Build history of the part. All positions in model axes, mm. Give positions to 0.01 mm unless a question says otherwise; leave off trailing zeros. Loops run counter-clockwise (first coordinate to the right, second up) from the corner with the lowest first, then second, coordinate; pieces in that order, holes last. Notation, with made-up numbers: M -13,6.5 L 20,6.5 A23 ccw 20,14.5 Z; hole C 89.5,-14 d8. An arc over 180 degrees is marked long. Answer as a JSON object with one key per item and string values. Group by question number.
1. Slice it at C-C (y = -11). List the corners of the cut face in (x, z), then the cut area to 3 significant figures.
2. Slice it at A-A (x = 0). List the corners of the cut face in (y, z), then the cut area to 3 significant figures.
3. Drop flat-ended pins along their axis: pin 1 Ø2 at (y, z) = (0.5, 2) entering from +X; pin 2 Ø2 at (y, z) = (-28, 4) entering from +X; pin 3 Ø3 at (x, y) = (-13, 36) entering from +Z; pin 4 Ø3 at (y, z) = (-46, 1) entering from -X. Give the stop position or say it passes through.
4. Slice it at D-D (y = -45). List the corners of the cut face in (x, z), then the cut area to 3 significant figures.
5. Slice it at B-B (z = 5.1). List the corners of the cut face in (x, y).
6. Drill centre lines: line 1 along Y through (x, z) = (0, 3.4); line 2 along Y through (x, z) = (7.5, 0.25); line 3 along X through (y, z) = (-31.5, 2.9). Where is each one in solid material? Low to high. Write a range as [from, to].
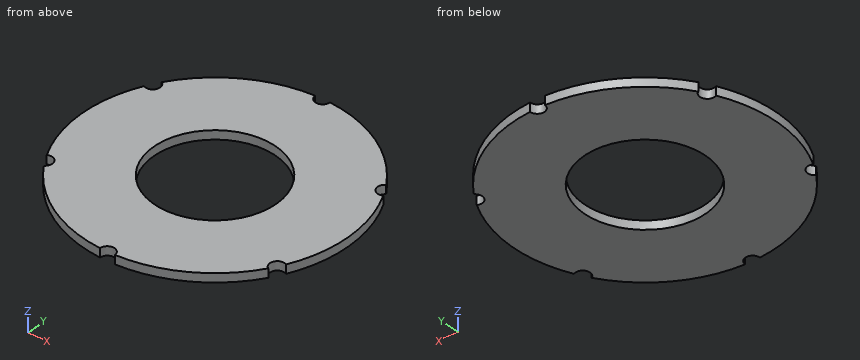
from build123d import *

# Parameters (mm, degrees)
SKETCH1_R                  = 90
SKETCH1_R_2                = 41.5
BOSS_EXTRUDE1_DEPTH        = 6
F_10_0MM_DOWEL_HOLE1_D     = 10
F_10_0MM_DOWEL_HOLE1_DEPTH = 9.906
F_10_0MM_DOWEL_HOLE1_TIP   = 3.004303095


with BuildPart() as part:
    # Sketch1 → Boss-Extrude1 (new body)
    with BuildSketch(Plane.XY):
        Circle(SKETCH1_R)
        Circle(SKETCH1_R_2, mode=Mode.SUBTRACT)
    extrude(amount=BOSS_EXTRUDE1_DEPTH)

    # Ø10.0mm Dowel Hole1
    with Locations(Plane(origin=(0, 0, 0), x_dir=(-1, 0, 0), z_dir=(0, 0, -1))):
        with Locations((-77.942286341, 45), (-77.942286341, -45), (0, -90), (77.942286341, -45), (77.942286341, 45), (0, 90)):
            Hole(F_10_0MM_DOWEL_HOLE1_D / 2, depth=F_10_0MM_DOWEL_HOLE1_DEPTH)
            with Locations((0, 0, -(F_10_0MM_DOWEL_HOLE1_DEPTH + F_10_0MM_DOWEL_HOLE1_TIP / 2))):  # 118° drill point
                Cone(0, F_10_0MM_DOWEL_HOLE1_D / 2, F_10_0MM_DOWEL_HOLE1_TIP, mode=Mode.SUBTRACT)


solid = part.part
Established:
{
 "1": {"outline": "M -89.33,0 L -40.02,0 L -40.02,6 L -89.33,6 Z; M 40.02,0 L 89.33,0 L 89.33,6 L 40.02,6 Z", "area": "592 mm^2"},
 "2": {"outline": "M -85,0 L -41.5,0 L -41.5,6 L -85,6 Z; M 41.5,0 L 85,0 L 85,6 L 41.5,6 Z", "area": "522 mm^2"},
 "3": {"pin 1": "stops at x = 90", "pin 2": "stops at x = 85.85", "pin 3": "passes through", "pin 4": "stops at x = -73.61"},
 "4": {"outline": "M -72.94,0 L 72.94,0 L 72.94,6 L -72.94,6 Z", "area": "875 mm^2"},
 "5": {"outline": "M -80.32,-40.6 A5 cw -75.32,-49.26 A90 ccw -5,-89.86 A5 cw 5,-89.86 A90 ccw 75.32,-49.26 A5 cw 80.32,-40.6 A90 ccw 80.32,40.6 A5 cw 75.32,49.26 A90 ccw 5,89.86 A5 cw -5,89.86 A90 ccw -75.32,49.26 A5 cw -80.32,40.6 A90 ccw Z; hole C 0,0 d83"},
 "6": {"line 1": "y = [-85, -41.5], [41.5, 85]", "line 2": "y = [-89.69, -40.82], [40.82, 89.69]", "line 3": "x = [-84.31, -27.02], [27.02, 84.31]"}
}
